from build123d import *

# Parameters (mm, degrees)
PAD_DEPTH     = 3.4
FILLET_R      = 4
SKETCH001_R   = 18
SKETCH001_R_2 = 6.25
PAD001_DEPTH  = 36
SKETCH002_W   = 12
SKETCH002_H   = 42
SKETCH002_R   = 2.65
PAD002_DEPTH  = 48
FILLET002_R   = 2


with BuildPart() as part:
    # Sketch → Pad (new body)
    with BuildSketch(Plane.XY):
        with BuildLine():
            Line((-65, 0), (-65, -60))
            Line((-65, -60), (65, -60))
            Line((65, -60), (65, 0))
            ThreePointArc((65, 0), (0, 45.409517), (-65, 0))
        make_face()
    extrude(amount=PAD_DEPTH)

    # Fillet
    fillet_edges = [part.edges().sort_by_distance(p)[0] for p in [
        (65, -60, 1.7),
        (-65, -60, 1.7),
    ]]
    fillet(fillet_edges, radius=FILLET_R)

    # Sketch001 (on Face6 of Pad) → Pad001 (join)
    with BuildSketch(Plane.XY.offset(3.4)):
        with Locations((42, -6)):
            Circle(SKETCH001_R)
        with Locations((42, -6)):
            Circle(SKETCH001_R_2, mode=Mode.SUBTRACT)
    pad001 = extrude(amount=PAD001_DEPTH)

    # Mirrored: Pad001 across YZ
    add(pad001.mirror(Plane.YZ))

    # Sketch002 (on Face5 of Mirrored) → Pad002 (join)
    with BuildSketch(Plane.XY.offset(3.4)):
        with Locations((-27.4, -35)):
            Rectangle(SKETCH002_W, SKETCH002_H)
        with Locations((-27.4, -26)):
            Circle(SKETCH002_R, mode=Mode.SUBTRACT)
        with Locations((-27.4, -44)):
            Circle(SKETCH002_R, mode=Mode.SUBTRACT)
    pad002 = extrude(amount=PAD002_DEPTH)

    # Mirrored001: Pad002 across Sketch002 V_Axis
    add(pad002.mirror(Plane(origin=(0, 0, 3.4), x_dir=(0, 0, 1), z_dir=(1, 0, 0))))

    # Fillet002
    fillet002_edges = [part.edges().sort_by_distance(p)[0] for p in [
        (33.4, -14, 45.4),
        (-33.4, -14, 45.4),
    ]]
    fillet(fillet002_edges, radius=FILLET002_R)


solid = part.part
Design review of the part built by this model. Coordinates are the model's own, in mm. A direction names the side the tool comes from. Give positions to 0.01 mm unless a question says otherwise; leave off trailing zeros. Write each loop counter-clockwise with the first axis right and the second up, starting at its lowest first coordinate (ties: lowest second). Pieces come first, ordered by that corner, then holes. Notation, with made-up numbers: M 9,14 L 48,14 A23 ccw 48,27 Z; hole C 66.25,-10.5 d9. An arc over 180 degrees is marked long. Answer as a JSON object with one key per item and string values. Group by question number.
1) We need section D-D (x = 27.4). Give the boundary of the cut face in (y, z).
2) We need section C-C (z = 26.5). Give the boundary of the cut face in (x, y), and give its area (3 significant figures).
3) Mouldability with a two-part tool opening along Y and no side actions: class faces 4 (the face through (-1, -60, 2)), 5 (the face through (27, -44, 3.4)), 6 (the face through (-21.4, -35, 27)) as released by +Y, released by -Y, zero draft, split by the parting line, or undercut.
4) We need section B-B (y = -44). Give the boundary of the cut face in (x, z).
5) We need section A-A (z = 45). Give the boundary of the cut face in (x, y).
6) For line 1 along Y through (x, z) = (-42, 27); line 2 along Y through (x, z) = (-27, 30); line 3 along X through (y, z) = (-0.5, 30), list the stretches that pass through material, from the lowest coordinate up.
7) Tool access review of faces 1 (the face through (27, -35, 51.4)), 2 (the face through (-24.95, -27.01, 27.06)), 3 (the face through (-50, -6, 39.4)): name each direction out of +Z, -Z, +X, -X, +Y, -Y from which nothing blocks a thin tool from reaching the whole face with its end or side.
8) Clearance check with flat-ended pins moving along their axes: pin 1 Ø16 at (x, y) = (-42, -6) entering from +Z; pin 2 Ø8.5 at (x, y) = (27.4, -26) entering from +Z; pin 3 Ø8 at (x, z) = (24, 39) entering from +Y; pin 4 Ø6 at (y, z) = (-19.5, 20) entering from -X. State where each tip first meets the part, or that it passes through.
Answer key:
{
 "1": {"outline": "M -60,0 L 39.76,0 L 39.76,3.4 L 4.53,3.4 L 4.53,39.4 L -14,39.4 L -14,51.4 L -23.35,51.4 L -23.35,3.4 L -28.65,3.4 L -28.65,51.4 L -41.35,51.4 L -41.35,3.4 L -46.65,3.4 L -46.65,51.4 L -56,51.4 L -56,3.4 L -60,3.4 Z"},
 "2": {"outline": "M -33.4,-56 L -21.4,-56 L -21.4,-14 L -25.88,-14 A18 ccw long -33.4,-21.81 Z; M 21.4,-56 L 33.4,-56 L 33.4,-21.81 A18 ccw long 25.88,-14 L 21.4,-14 Z; hole C -42,-6 d12.5; hole C -27.4,-44 d5.3; hole C -27.4,-26 d5.3; hole C 27.4,-44 d5.3; hole C 27.4,-26 d5.3; hole C 42,-6 d12.5", "area": "2,640 mm²"},
 "3": {"face 4": "released by -Y", "face 5": "undercut", "face 6": "zero draft"},
 "4": {"outline": "M -65,0 L 65,0 L 65,3.4 L 33.4,3.4 L 33.4,51.4 L 30.05,51.4 L 30.05,3.4 L 24.75,3.4 L 24.75,51.4 L 21.4,51.4 L 21.4,3.4 L -21.4,3.4 L -21.4,51.4 L -24.75,51.4 L -24.75,3.4 L -30.05,3.4 L -30.05,51.4 L -33.4,51.4 L -33.4,3.4 L -65,3.4 Z"},
 "5": {"outline": "M -33.4,-56 L -21.4,-56 L -21.4,-14 L -31.4,-14 A2 ccw -33.4,-16 Z; M 21.4,-56 L 33.4,-56 L 33.4,-16 A2 ccw 31.4,-14 L 21.4,-14 Z; hole C -27.4,-44 d5.3; hole C -27.4,-26 d5.3; hole C 27.4,-44 d5.3; hole C 27.4,-26 d5.3"},
 "6": {"line 1": "y = -24 to -12.25, 0.25 to 12", "line 2": "y = -56 to -46.62, -41.38 to -28.62, -23.38 to 3.95", "line 3": "x = -59.14 to -44.97, -39.03 to -24.86, 24.86 to 39.03, 44.97 to 59.14"},
 "7": {"face 1": "+Z, +X, -X, +Y, -Y", "face 2": "+Z", "face 3": "+Z, -X, +Y"},
 "8": {"pin 1": "stops at z = 39.4", "pin 2": "stops at z = 51.4", "pin 3": "stops at y = 5.31", "pin 4": "stops at x = -56.62"}
}
